Autodesk Inventor part; units mm, degrees
ref_plane "YZ Plane" through (0, 0, 0) normal (1, 0, 0) x (0, 1, 0)
ref_plane "XZ Plane" through (0, 0, 0) normal (0, 1, 0) x (-1, 0, 0)
ref_plane "XY Plane" through (0, 0, 0) normal (0, 0, 1) x (1, 0, 0)
sketch "スケッチ1" plane through (0, 0, 0) normal (0, 0, 1) x (1, 0, 0)
  line L0 (-16, 21.5) -> (-10.583, 21.5) construction
  line L1 (16, 21.5) -> (16, 9.5) construction
  line L2 (16, -21.5) -> (-16, -21.5)
  line L3 (-16, -21.5) -> (-16, 9.5)
  line L4 (-16, 21.5) -> (16, -21.5) construction
  line L5 (16, 21.5) -> (-16, -21.5) construction
  line L6 (-14.4, -21.5) -> (-14.4, -30)
  line L7 (-14.4, -30) -> (14.4, -30)
  line L8 (0, 21.5) -> (0, -21.5) construction
  line L9 (14.4, -21.5) -> (14.4, -30)
  line L10 (-13.5, 21.5) -> (-13.5, -21.5) construction
  circle A0 centre (0, 9.5) radius 6
  circle A1 centre (0, 9.5) radius 4
  arc A2 (-10.583, 21.5) -> (-16, 9.5) centre (0, 9.5) ccw
  arc A3 (16, 9.5) -> (10.583, 21.5) centre (0, 9.5) ccw
  line L11 (-10.583, 21.5) -> (10.583, 21.5)
  line L12 (-16, 9.5) -> (-16, 21.5) construction
  line L13 (10.583, 21.5) -> (16, 21.5) construction
  line L14 (16, 9.5) -> (16, -21.5)
  circle A4 centre (0, 9.5) radius 3
  circle A5 centre (0, 9.5) radius 4.8
  point P0 (0, 0)
  point P1 (-13.5, 8.5)
  point P2 (-13.5, -18.5)
  point P3 (13.5, 8.5)
  point P4 (13.5, -18.5)
  dimension "d0" = 32
  dimension "d1" = 43
  dimension "d4" = 28.8
  dimension "d5" = 8.5
  dimension "d8" = 27
  dimension "d9" = 8.5
  dimension "d12" = 18.5
  dimension "d13" = 12
  dimension "d14" = 8
  dimension "d15" = 9.5
  dimension "d17" = 16
  dimension "d32" = 13.5
  dimension "d47" = 6
  dimension "d67" = 9.6
extrude "押し出し1" add sketch "スケッチ1" against normal blind 12.2 contours L2 L3 A2 L11 A3 L14 | A0 | A1 | A4 | A5
extrude "押し出し2" add sketch "スケッチ1" against normal blind 12 contours L9 L7 L6 L2
extrude "押し出し3" add sketch "スケッチ1" against normal blind 14 contours A0 | A1 | A4 | A5
extrude "押し出し4" add sketch "スケッチ1" against normal blind 17.7 contours A1 | A4
chamfer "面取り1" distance 1.2 angle 45 1 edges at (-6, 9.5, -14)
sketch "スケッチ2" plane through (0, 9.5, -17.7) normal (0, 0, -1) x (-1, 0, 0)
  circle A0 centre (0, 0) radius 4
  point P0 (0, -9.5)
hole "穴1" at (0, 9.5, -17.7) direction (0, 0, 1) diameter 2.459 depth 6
extrude "押し出し5" add sketch "スケッチ1" along normal blind 20.3 contours L2 L3 A2 L11 A3 L14 | A0 | A1 | A4 | A5
hole "穴2" at (-13.5, 8.5, 0) at (-13.5, -18.5, 0) at (13.5, 8.5, 0) at (13.5, -18.5, 0) direction (0, 0, 1) diameter 2.7 end through all both
extrude "押し出し6" cut sketch "スケッチ1" against normal blind 0.4 contours L9 L7 L6 L2
fillet "フィレット1" radius 2 2 edges at (16, -21.5, 4.05) (-16, -21.5, 4.05)
extrude "押し出し7" add sketch "スケッチ1" along normal blind 21.2 contours A0 | A1 | A4 | A5
extrude "押し出し8" add sketch "スケッチ1" along normal blind 23.75 contours A4
sketch "スケッチ3" plane through (0, 9.5, 23.75) normal (0, 0, 1) x (1, 0, 0)
  circle A0 centre (0, 0) radius 1.2295
  point P0 (0, -9.5)
hole "穴3" at (0, 9.5, 23.75) direction (0, 0, -1) diameter 2.459 end through all
sketch "スケッチ4" plane through (0, 9.5, 21.2) normal (0, 0, 1) x (1, 0, 0)
  circle A0 centre (0, 0) radius 4
  circle A1 centre (0, 0) radius 3
  point P0 (0, -9.5)
extrude "押し出し9" cut sketch "スケッチ4" against normal blind 2.3
chamfer "面取り2" distance 0.5 angle 45 1 edges at (-3, 9.5, 23.75)
extrude "押し出し10" add sketch "スケッチ1" against normal blind 14.2 contours A5
chamfer "面取り4" distance 0.1 angle 45 2 edges at (-4, 9.5, 21.2) (-6, 9.5, 21.2)
properties part number "B3M-SC-1040-A"
Source: CAD feature listing. Evaluate the final solid. Frame: model axes, mm. A direction names the side the tool comes from. Round coordinates to 2 decimals unless told otherwise and drop trailing zeros. Loops run counter-clockwise (first coordinate to the right, second up) from the corner with the lowest first, then second, coordinate; pieces in that order, holes last.
Q1. Section C-C, the plane y = -13. Return loops of the section in (x, z).
Q2. Ray query, line 1 (X direction, y = -18.5, z = -3); line 2 (Y direction, x = 13, z = 9); line 3 (Y direction, x = 13.5, z = 14). Return the intervals inside material, ascending.
Q3. Access query for faces 4 (the face through (3.815, 10.701, -15.926)), 5 (the face through (-0.78, 3.55, 20.69)), 6 (the face through (1, 11, 23.75)), 7 (the face through (0, -26, -0.4)). Directions: +Z, -Z, +X, -X, +Y, -Y. A direction counts if a zero-diameter tool reaches every point of the face in a straight line with its end or side. Return the directions, or none.
Q4. Section A-A, the plane z = -3. Return loops of the section in (x, y).
Q5. Section B-B, the plane x = 9.5. Return loops of the section in (y, z).
Q6. First-contact query: P1, Ø3, axis at y = 16, z = 11, coming from the -X side; P2, Ø5, axis at x = -5.5, y = 6, coming from the +Z side; P3, Ø1, axis at x = 2, y = 0, coming from the +Z side. Flat tips, straight axial feed; report the tip coordinate or a pass-through.
Q7. Mould query, pull axis X, two halves, no side actions, for faces 1 (the face through (-3, 11, 18.9)), 2 (the face through (-14.4, -26, -6)), 3 (the face through (0, -21.5, 10)). Classes: pulls with the +X half, pulls with the -X half, needs draft (parallel to the pull), parting line crosses it, or undercut.
Q8. Section D-D, the plane z = 6. Return loops of the section in (x, y).
Solutions:
1. outline: (-16, -12.2) - (16, -12.2) - (16, 20.3) - (-16, 20.3) - close
2. line 1: x = -16 to -14.85, -12.15 to 12.15, 14.85 to 16
2. line 2: y = -21.5 to -19.75, -17.25 to 7.25, 9.75 to 18.83
2. line 3: y = -21.5 to -19.85, -17.15 to 7.15, 9.85 to 18.09
3. face 4: -Z
3. face 5: +Z
3. face 6: +Z, +X, -X, +Y, -Y
3. face 7: +Z, +X, -X, -Y
4. outline: (-16, -19.5) arc R2 ccw to (-14.4, -21.46) - (-14.4, -30) - (14.4, -30) - (14.4, -21.46) arc R2 ccw to (16, -19.5) - (16, 9.5) arc R16 ccw to (10.58, 21.5) - (-10.58, 21.5) arc R16 ccw to (-16, 9.5) - close; hole circle Ø2.7 at (-13.5, -18.5); hole circle Ø2.7 at (-13.5, 8.5); hole circle Ø2.46 at (0, 9.5); hole circle Ø2.7 at (13.5, -18.5); hole circle Ø2.7 at (13.5, 8.5)
5. outline: (-30, -12) - (-21.5, -12) - (-21.5, -12.2) - (21.5, -12.2) - (21.5, 20.3) - (-21.5, 20.3) - (-21.5, -0.4) - (-30, -0.4) - close
6. P1: stops at x = -15.2
6. P2: stops at z = 21.2
6. P3: stops at z = 20.3
7. face 1: undercut
7. face 2: pulls with the -X half
7. face 3: needs draft
8. outline: (-16, -19.5) arc R2 ccw to (-14, -21.5) - (14, -21.5) arc R2 ccw to (16, -19.5) - (16, 9.5) arc R16 ccw to (10.58, 21.5) - (-10.58, 21.5) arc R16 ccw to (-16, 9.5) - close; hole circle Ø2.7 at (-13.5, -18.5); hole circle Ø2.7 at (-13.5, 8.5); hole circle Ø2.46 at (0, 9.5); hole circle Ø2.7 at (13.5, -18.5); hole circle Ø2.7 at (13.5, 8.5)
